```python
from build123d import *

# Parameters (mm, degrees)
SKETCH001_W   = 30
SKETCH001_H   = 30
SKETCH001_W_2 = 26
SKETCH001_H_2 = 26
PAD001_DEPTH  = 560


with BuildPart() as part:
    # Sketch001 → Pad001 (new body)
    with BuildSketch(Plane.XZ):
        with Locations((15, -15)):
            Rectangle(SKETCH001_W, SKETCH001_H)
        with Locations((15, -15)):
            Rectangle(SKETCH001_W_2, SKETCH001_H_2, mode=Mode.SUBTRACT)
    extrude(amount=PAD001_DEPTH)


with BuildPart() as part_1:
    # Body001 placement: moved
    add(part.part.moved(Location((-240, 390, 0))))


solid = part_1.part
```
Geometry check sheet. Reference: the model listing, model coordinates, mm. A direction names the side the tool comes from. Give positions to 0.01 mm unless a question says otherwise; leave off trailing zeros. Order: outer loops, then holes, each group sorted by start corner. A loop starts at its lowest first (then second) coordinate and runs counter-clockwise, first axis right, second up.
1. Section check C-C, the plane y = -36. Enter the section's corners in (x, z), and give its area (3 significant figures).
2. Thickness scan on L1, parallel to Z at x = -224.25, y = 361.5; L2, parallel to X at y = 244.5, z = -23. Record the ranges inside material, lowest first.
3. Section check B-B, the plane x = -227. Enter the section's corners in (y, z), and give its area (3 significant figures).
4. Release check for a two-part mould opening along Z. For faces 3 (the face through (-225, 114, -30)), 4 (the face through (-210, 114, -15)), 5 (the face through (-225, 114, -2)) record: pulls with the +Z half, pulls with the -Z half, needs draft (parallel to the pull), parting line crosses it, or undercut.
5. Section check A-A, the plane z = -14.75. Enter the section's corners in (x, y).
6. Access from +Z, -Z, +X, -X, +Y, -Y to the whole of each face (thin tool, end or side, straight path). Record for faces 1 (the face through (-225, 114, -28)), 2 (the face through (-225, 114, 0)).
Values follow:
1. outline: (-240, -30) - (-210, -30) - (-210, 0) - (-240, 0) - close; hole (-238, -28) - (-212, -28) - (-212, -2) - (-238, -2) - close
1. area: 224 mm2
2. L1: z = -30 to -28, -2 to 0
2. L2: x = -240 to -238, -212 to -210
3. outline: (-170, -30) - (390, -30) - (390, -28) - (-170, -28) - close; (-170, -2) - (390, -2) - (390, 0) - (-170, 0) - close
3. area: 2,240 mm2
4. face 3: pulls with the -Z half
4. face 4: needs draft
4. face 5: undercut
5. outline: (-240, -170) - (-238, -170) - (-238, 390) - (-240, 390) - close; (-212, -170) - (-210, -170) - (-210, 390) - (-212, 390) - close
6. face 1: +Y, -Y
6. face 2: +Z, +X, -X, +Y, -Y
